Autodesk Inventor part; units mm, degrees
ref_plane "Work Plane1" through (173.3333, 20, -7) normal (1, 0, 0) x (0, 0, -1)
ref_plane "Work Plane2" through (86.6667, 20, -7) normal (1, 0, 0) x (0, 0, -1)
ref_plane "YZ Plane" through (0, 0, 0) normal (1, 0, 0) x (0, 1, 0)
sketch "Sketch1" plane through (0, 0, 0) normal (0, 0, 1) x (1, 0, 0)
  line L0 (0, 0) -> (260, 0)
  line L1 (260, 0) -> (260, 20)
  line L2 (260, 20) -> (0, 20)
  line L3 (0, 20) -> (0, 0)
  dimension "d0" = 260
  dimension "d1" = 20
extrude "Extrusion1" add sketch "Sketch1" along normal blind 3
sketch "Sketch2" plane through (0, 0, 0) normal (0, 0, -1) x (-1, 0, 0)
  line L0 (0, 0) -> (-260, 0)
  line L1 (-12.5251, -24.7625) -> (-37.9251, -24.7625)
  line L2 (-260, 20) -> (0, 20)
  point P0 (-25.2251, 30)
  dimension "d5" = 25.4
  dimension "d6" = 12.7
  dimension "d62" = 10
sketch "Sketch5" plane through (0, 0, 0) normal (-1, 0, 0) x (0, 0, 1)
  line L0 (0, 20) -> (3, 20)
  line L1 (3, 20) -> (-7, 20)
  line L2 (-7, 20) -> (-7, 40)
  line L3 (-7, 40) -> (3, 40)
  line L4 (3, 40) -> (3, 20)
  point P0 (0, 0)
  point P1 (3, 30)
  point P2 (1.5, 20)
  dimension "d31" = 10
  dimension "d32" = 20
extrude "Extrusion3" add sketch "Sketch5" against normal up to surface (260 mm away)
sketch "Sketch6" plane through (0, 0, 3) normal (0, 0, 1) x (1, 0, 0)
  line L0 (0, 0) -> (0, 40)
  line L1 (260, 0) -> (260, 40)
  line L2 (0, 40) -> (260, 40)
  point P0 (42.6875, 30)
  point P1 (77.6125, 30)
  point P2 (182.3875, 30)
  point P3 (217.3125, 30)
  point P4 (112.5375, 30)
  point P5 (147.4625, 30)
  dimension "d35" = 42.6875
  dimension "d46" = 42.6875
  dimension "d47" = 34.925
  dimension "d48" = 34.925
  dimension "d49" = 34.925
  dimension "d50" = 34.925
  dimension "d51" = 10
hole "Hole2" at (42.6875, 30, 3) at (77.6125, 30, 3) at (182.3875, 30, 3) at (217.3125, 30, 3) at (112.5375, 30, 3) at (147.4625, 30, 3) direction (0, 0, -1) diameter 6 end through all
hole "Hole3" at (25.2251, 30, 0) direction (0, 0, 1) diameter 4.3 depth 6
pattern_linear "Rectangular Pattern2" count 7 spacing 34.925 along (1, 0, 0) of "Hole3"
chamfer "Chamfer1" distance 2 angle 45 1 edges at (130, 20, 0)
sketch "Sketch7" plane through (0, 0, 0) normal (-1, 0, 0) x (0, 0, 1)
  line L0 (0, 0) -> (3, 0)
  line L1 (0, 0) -> (3.6796, 0)
  line L2 (3.6796, 0) -> (3.6796, 5)
  line L3 (3.6796, 5) -> (0, 5)
  line L4 (0, 5) -> (0, 0)
  dimension "d66" = 5
extrude "Extrusion4" cut sketch "Sketch7" against normal through all
ref_plane "Work Plane1" through (173.3333, 20, -7) normal (1, 0, 0) x (0, 0, -1)
ref_plane "Work Plane2" through (86.6667, 20, -7) normal (1, 0, 0) x (0, 0, -1)
sketch "Sketch8" plane through (173.3333, 20, -7) normal (1, 0, 0) x (0, 0, -1)
  line L0 (-10, -15) -> (-7, -15)
  line L1 (-7, -15) -> (-7, -2)
  line L2 (-5, 0) -> (-7, -2)
  line L3 (0, 0) -> (-5, 0)
  line L4 (0, 20) -> (0, 0)
  line L5 (-10, 20) -> (0, 20)
  line L6 (-10, -15) -> (-10, 20)
  point P0 (-7, -20)
extrude "Extrusion5" cut sketch "Sketch8" against normal through all
properties part number "IR_Mount_Plate_3DPrint"
Verification items for the finished model (mm, model axes). A direction names the side the tool comes from. Give positions to 0.01 mm unless a question says otherwise; leave off trailing zeros. Order: outer loops, then holes, each group sorted by start corner. A loop starts at its lowest first (then second) coordinate and runs counter-clockwise, first axis right, second up. Notation, with made-up numbers: M 63,-7.5 L 94,-7.5 A11 cw 94,0.5 Z; hole C -3,-21 d5. An arc over 180 degrees is marked long. Return JSON: item names as keys, results as strings. Group by question number.
1) Section check C-C on x = 207. Record the cut outline in (y, z).
2) Mould release check, pull along X, two halves, no side actions. Record for faces 4 (the face through (200, 30, 0)), 5 (the face through (216, 25, -7)), 6 (the face through (173.333, 27, -1)): pulls with the +X half, pulls with the -X half, needs draft (parallel to the pull), parting line crosses it, or undercut.
3) Section check B-B on z = 1.75. Record the cut outline in (x, y), and give its area (3 significant figures).
4) Section check A-A on y = 30. Record the cut outline in (x, z), and give its area (3 significant figures).
5) Access from +Z, -Z, +X, -X, +Y, -Y to the whole of each face (thin tool, end or side, straight path). Record for faces 1 (the face through (260, 26, -1)), 2 (the face through (216, 20, -4)), 3 (the face through (232.962, 31.156, 1.521)).
6) Go/stop test with flat-tipped pins: pin 1 Ø9.5 at (x, y) = (182.39, 30) entering from -Z; pin 2 Ø1.5 at (x, z) = (241.5, -4) entering from -Y; pin 3 Ø1.5 at (x, z) = (223, -2.5) entering from -Y; pin 4 Ø12 at (x, y) = (244, 10.5) entering from -Z. Record where each tip stops, or that it passes through.
7) Scan lines: line 1 (X direction, y = 30, z = -4); line 2 (X direction, y = 30, z = 1.25); line 3 (X direction, y = 31, z = -1.5). Record each from-to range of solid material in increasing order.
8) Section check D-D on z = -4.25. Record the cut outline in (x, y), and give its area (3 significant figures).
Answer block:
{
 "1": {"outline": "M 5,0 L 18,0 L 20,-2 L 20,-7 L 40,-7 L 40,3 L 5,3 Z"},
 "2": {"face 4": "undercut", "face 5": "needs draft", "face 6": "pulls with the -X half"},
 "3": {"outline": "M 173.33,5 L 260,5 L 260,40 L 173.33,40 Z; hole C 182.39,30 d6; hole C 199.85,30 d4.3; hole C 217.31,30 d6; hole C 234.78,30 d4.3", "area": "2,950 mm^2"},
 "4": {"outline": "M 173.33,-7 L 179.39,-7 L 179.39,3 L 173.33,3 Z; M 185.39,-7 L 214.31,-7 L 214.31,3 L 202,3 L 202,0 L 197.7,0 L 197.7,3 L 185.39,3 Z; M 220.31,-7 L 260,-7 L 260,3 L 236.93,3 L 236.93,0 L 232.63,0 L 232.63,3 L 220.31,3 Z", "area": "721 mm^2"},
 "5": {"face 1": "+Z, -Z, +X, +Y, -Y", "face 2": "-Z, +X, -X, -Y", "face 3": "+Z"},
 "6": {"pin 1": "stops at z = -7", "pin 2": "stops at y = 20", "pin 3": "stops at y = 19.75", "pin 4": "stops at z = 0"},
 "7": {"line 1": "x = 173.33 to 179.39, 185.39 to 214.31, 220.31 to 260", "line 2": "x = 173.33 to 179.39, 185.39 to 197.7, 202 to 214.31, 220.31 to 232.63, 236.93 to 260", "line 3": "x = 173.33 to 179.56, 185.22 to 214.48, 220.14 to 260"},
 "8": {"outline": "M 173.33,20 L 260,20 L 260,40 L 173.33,40 Z; hole C 182.39,30 d6; hole C 217.31,30 d6", "area": "1,680 mm^2"}
}
